Could you check a few things on this model? Use its own coordinates, in mm. Face numbers are marked on the shaded views. A direction names the side the tool comes from. Give positions to 0.01 mm unless a question says otherwise; leave off trailing zeros. Write each loop counter-clockwise with the first axis right and the second up, starting at its lowest first coordinate (ties: lowest second). Pieces come first, ordered by that corner, then holes. Notation, with made-up numbers: M 71,76 L 122,76 A18 ccw 122,93 Z; hole C 76.5,18 d11. An arc over 180 degrees is marked long. Answer as CSV lines item,"result". Start each with the question number.
from build123d import *

# Parameters (mm, degrees)
F2_DEPTH = 162.56
F1_R     = 87.2293400051
F5_DEPTH = 157.48
F7_DEPTH = 157.48
F9_DEPTH = 157.48


with BuildPart() as f2:
    # F0 (on Front) → F2 (new body)
    with BuildSketch(Plane.XZ):
        Polygon((-3.7715153303, 16.7024247348), (2.6939406525, 35.8293950558), (-36.9069688022, 38.2539406419), (-21.2821215391, 11.8533335626), align=None)
    extrude(amount=F2_DEPTH)


with BuildPart() as f2b:
    # F1 (on Front) → F2, piece 2 (new body)
    with BuildSketch(Plane.XZ):
        Circle(F1_R)
    extrude(amount=F2_DEPTH)

    # F4 (on face) → F5 (cut)
    with BuildSketch(Plane(origin=(0, 0, 0), x_dir=(-1, 0, 0), z_dir=(0, 1, 0))):
        Polygon((-26.3271015137, 45.3784566633), (-52.4583123624, 11.8539193645), (-39.796795696, 2.6937914081), (-26.3271015137, 12.3927500099), align=None)
    extrude(amount=-F5_DEPTH, mode=Mode.SUBTRACT)

    # F6 (on face) → F7 (cut)
    with BuildSketch(Plane(origin=(0, 0, 0), x_dir=(-1, 0, 0), z_dir=(0, 1, 0))):
        Polygon((-12.5880083069, 17.781060189), (10.3104757145, 45.3784566633), (53.9522953331, 53.074490279), (-10.1634636521, 70.0476691127), align=None)
        Polygon((50.9889610112, -17.2429550439), (23.5107783228, 24.7858650982), (13.2738091052, -17.2429550439), align=None)
        Polygon((73.3486637473, 20.4752162099), (61.4953264594, 34.7542390227), (42.0989617705, 11.8539193645), (57.5345901374, 4.2026060604), (64.728051424, 12.3927500099), (64.728051424, 13.7398280203), (74.6956318617, 8.3515178412), align=None)
        Polygon((-17.7064947784, -24.2477599531), (-19.8616459966, -22.6312670857), (-50.3031611443, -39.6044403315), (21.0862327367, -65.7377541065), (13.2738091052, -39.6044403315), align=None)
    extrude(amount=-F7_DEPTH, mode=Mode.SUBTRACT)

    # F8 (on face) → F9 (cut)
    with BuildSketch(Plane(origin=(0, 0, 0), x_dir=(-1, 0, 0), z_dir=(0, 1, 0))):
        Polygon((-48.995775217, 47.9173291132), (-65.1198253036, 32.3294997215), (-77.2425532341, 5.3879469633), (-70.7771033049, -40.9515202045), (-28.4822527319, -15.6264640391), (-54.8828579485, 2.1549605299), align=None)
        Polygon((-23.902554065, 60.1852526106), (-23.902554065, 63.8511106372), (-40.3355844319, 51.4579974115), (-26.0577071458, 48.7638451159), align=None)
        Polygon((63.6504739523, -52.2669777274), (56.9156296551, -28.0195791274), (47.2174473107, -52.2669777274), align=None)
    extrude(amount=-F9_DEPTH, mode=Mode.SUBTRACT)


solid = f2b.part
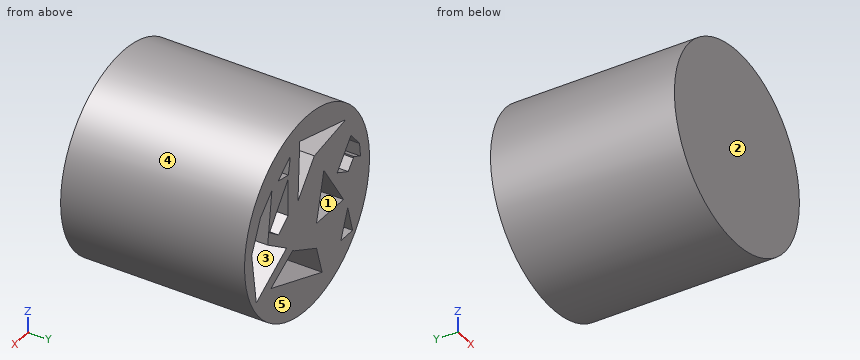
1. Will these pins go through, and if not, where does the flat tip stop? P1, Ø6, axis at x = -29, y = -48, coming from the -Z side; P2, Ø5, axis at x = -57.5, z = -46, coming from the +Y side; P3, Ø12, axis at x = 50, z = 64, coming from the +Y side; P4, Ø1.1, axis at y = -46, z = 13.5, coming from the +X side.
2. Imagine slicing it at A-A, the plane x = 0. Please give me the cut outline in (y, z).
3. On a 3-axis mill with a long thin cutter (end or side, diameter ignored), from which of +Z, -Z, +X, -X, +Y, -Y can I reach the whole of each face in a straight line? I mean the marked faces 1 and 2. Say none if no direction works.
4. Thinking about a two-plate mould opening in X: for the marked faces 3, 4 and 5, which applies, pulls with the +X half, pulls with the -X half, needs draft (parallel to the pull), parting line crosses it, or undercut?
5. Please list where these lines run through material, in increasing order: line 1 (X direction, y = -45, z = 38.5); line 2 (X direction, y = -152, z = 32); line 3 (X direction, y = -26.5, z = 33.5).
6. Imagine slicing it at C-C, the plane z = -33. Please give me the cut outline in (x, y).
7. Imagine slicing it at D-D, the plane x = 33.5. Please give me the cut outline in (y, z), plus the area to 3 significant figures.
8. Imagine slicing it at B-B, the plane y = -148.5. State how many separate pieces and enclosed holes the cut face has, plus the area to 3 significant figures.
Solutions:
1,P1,"z = -83.26"
1,P2,"y = -157.48"
1,P3,"y = 0"
1,P4,"x = 86.26"
2,outline,"M -162.56,-87.23 L 0,-87.23 L 0,-58.02 L -157.48,-58.02 L -157.48,-33.02 L 0,-33.02 L 0,32.95 L -157.48,32.95 L -157.48,67.36 L 0,67.36 L 0,87.23 L -162.56,87.23 Z"
3,face 1,"+Y"
3,face 2,"+Z, -Z, +X, -X, -Y"
4,face 3,"undercut"
4,face 4,"parting line crosses it"
4,face 5,"needs draft"
5,line 1,"-78.27 to -4.6, 11.63 to 26.33, 31.69 to 50.21, 58.74 to 78.27"
5,line 2,"-81.15 to -63.78, -59.16 to 0.79, 11.93 to 26.33, 36.76 to 51.04, 65.27 to 81.15"
5,line 3,"-80.54 to -62.54, -60.43 to -0.45, 11.86 to 26.33, 35.59 to 50.85, 63.91 to 80.54"
6,outline,"M -80.75,-162.56 L 80.75,-162.56 L 80.75,0 L 71.89,0 L 71.89,-157.48 L 57.5,-157.48 L 57.5,0 L 38.46,0 L 38.46,-157.48 L 0.05,-157.48 L 0.05,0 L -54.92,0 L -54.92,-157.48 L -58.3,-157.48 L -58.3,0 L -80.75,0 Z"
7,outline,"M -162.56,-80.54 L 0,-80.54 L 0,-45.76 L -157.48,-45.76 L -157.48,-30.24 L 0,-30.24 L 0,-18.63 L -157.48,-18.63 L -157.48,-12.25 L 0,-12.25 L 0,7.23 L -157.48,7.23 L -157.48,36.18 L 0,36.18 L 0,50.17 L -157.48,50.17 L -157.48,56.61 L 0,56.61 L 0,80.54 L -162.56,80.54 Z"
7,area,"17,200 mm²"
8,separate pieces,"1"
8,enclosed holes,"8"
8,area,"17,300 mm²"
